Autodesk Inventor part; units mm, degrees
ref_plane "YZ Plane" through (0, 0, 0) normal (1, 0, 0) x (0, 1, 0)
ref_plane "XZ Plane" through (0, 0, 0) normal (0, 1, 0) x (-1, 0, 0)
ref_plane "XY Plane" through (0, 0, 0) normal (0, 0, 1) x (1, 0, 0)
sketch "スケッチ1" plane through (0, 0, 0) normal (0, 1, 0) x (-1, 0, 0)
  line L0 (0, 0) -> (0, 10)
  line L1 (0, 0) -> (3.5, 0)
  line L2 (4, 0.5) -> (4, 3.5)
  line L3 (3.5, 4) -> (1.5, 4)
  line L4 (1.5, 4) -> (1.5, 10)
  line L5 (1.5, 10) -> (0, 10)
  line L6 (-0.8, 1.5) -> (0.8, 1.5)
  line L7 (0.8, 1.5) -> (0.8, 0)
  line L8 (0.8, 0) -> (-0.8, 0)
  line L9 (-0.8, 0) -> (-0.8, 1.5)
  line L10 (-0.8, 1.5) -> (0.8, 0) construction
  line L11 (0.8, 1.5) -> (-0.8, 0) construction
  line L12 (3.5, 0) -> (4, 0.5)
  line L13 (4, 3.5) -> (3.5, 4)
  point P0 (4, 0)
  point P1 (4, 4)
  point P2 (0, 0.75)
  dimension "d7" = 4
  dimension "d8" = 6
  dimension "d12" = 3
  dimension "d13" = 8
  dimension "d20" = 1.5
  dimension "d21" = 1.6
  dimension "d24" = 0.5
  dimension "d25" = 0.5
  dimension "d26" = 0.5
  dimension "d27" = 0.5
revolve "回転1" add sketch "スケッチ1" angle 360 about axis through (0, 0, 0) along (0, 0, 1) contours L0 L6 L7 L1 | L0 L5 L4 L3 L13 L2 L12 L1 L7 L6
thread "ねじ1"
extrude "押し出し1" cut sketch "スケッチ1" along normal through all both and the other way through all contours L8 L9 L6 L0 | L0 L6 L7 L1
properties part number "CSMKN-SUSTBS-M3-6" material "ステンレス鋼 AISI 304"
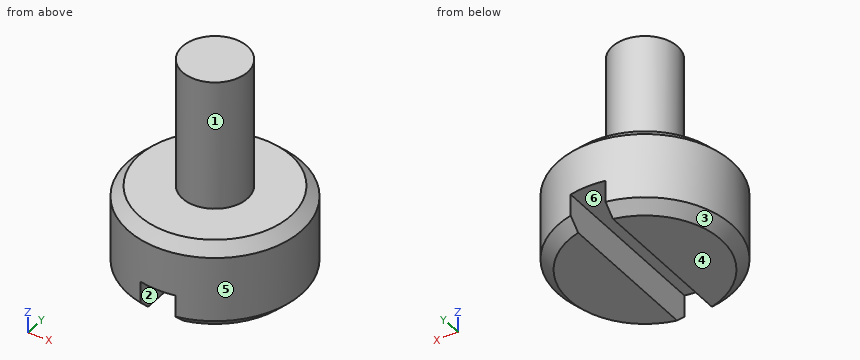
The listing builds one solid part. Answer for the finished solid, in the listing's coordinates (mm). Face numbers are marked on the shaded views. A direction names the side the tool comes from. Round coordinates to 2 decimals unless told otherwise and drop trailing zeros. Order: outer loops, then holes, each group sorted by start corner. A loop starts at its lowest first (then second) coordinate and runs counter-clockwise, first axis right, second up. Notation, with made-up numbers: (13, 6.5) - (54, 6.5) arc R11 cw to (54, 18.5) - close; hole circle Ø4 at (5, 75). An arc over 180 degrees is marked (long way). Write item = value, one per line. Start each with the question number.
1) For the marked faces 1, 2 and 3, determine the directions among +Z, -Z, +X, -X, +Y, -Y from which every point of the face is accessible in a straight line to the end or side of a thin tool.
2) Section D-D, the plane z = 3.25 is taken. Write down the section's boundary in (x, y).
3) For a pull along X with two mould halves and no side action, classify the marked faces 4, 5 and 6 as released by +X, released by -X, zero draft, split by the parting line, or undercut.
4) Section B-B, the plane x = 0 is taken. Write down the section's boundary in (y, z).
5) Section A-A, the plane y = 0 is taken. Write down the section's boundary in (x, z), plus the area to 3 significant figures.
6) Straight lines are drawn through the part: L1, parallel to Z at x = -3, y = 1; L2, parallel to Z at x = -0.5, y = 3; L3, parallel to X at y = -1, z = 9.75. For each, find the intervals that lie inside material, in ascending order.
7) Section C-C, the plane z = 1 is taken. Write down the section's boundary in (x, y).
8) Given pin 1 (1.2 mm diameter, centred on y = 1, z = 1, fed in from -X); pin 2 (0.5 mm diameter, centred on y = 0.5, z = 0.5, fed in from +X); pin 3 (1.5 mm diameter, centred on x = 1, z = 1.5, fed in from -Y), each flat-ended and moving along its own axis, determine where each tip first touches the part or whether it passes through.
Results list:
q1.face_1 = +Z
q1.face_2 = -Z, +Y, -Y
q1.face_3 = -Z, -X
q2.outline = circle Ø8 at (0, 0)
q3.face_4 = zero draft
q3.face_5 = split by the parting line
q3.face_6 = undercut
q4.outline = (-4, 1.5) - (4, 1.5) - (4, 3.5) - (3.5, 4) - (1.5, 4) - (1.5, 10) - (-1.5, 10) - (-1.5, 4) - (-3.5, 4) - (-4, 3.5) - close
q5.outline = (-4, 0.5) - (-3.5, 0) - (-0.8, 0) - (-0.8, 1.5) - (0.8, 1.5) - (0.8, 0) - (3.5, 0) - (4, 0.5) - (4, 3.5) - (3.5, 4) - (1.5, 4) - (1.5, 10) - (-1.5, 10) - (-1.5, 4) - (-3.5, 4) - (-4, 3.5) - close
q5.area = 47.1 mm^2
q6.L1 = 0 to 4
q6.L2 = 1.5 to 4
q6.L3 = -1.12 to 1.12
q7.outline = (-0.8, -3.92) - (-0.8, 3.92) arc R4 ccw to start; (0.8, -3.92) arc R4 ccw to (0.8, 3.92) - close
q8.pin_1 = -3.98
q8.pin_2 = 3.99
q8.pin_3 = -3.99
